Design review of the part built by this model. Coordinates are the model's own, in mm. A direction names the side the tool comes from. Coordinates: 2 decimals unless noted, no trailing zeros. Loops run counter-clockwise (first coordinate to the right, second up) from the corner with the lowest first, then second, coordinate; pieces in that order, holes last. Notation, with made-up numbers: M -21,2.25 L 30,2.25 A25 ccw 30,26.25 Z; hole C -13.75,83 d9. An arc over 180 degrees is marked long. Put each result on its own line as item: value. Start each with the question number.
(1) Clearance check with a flat-ended pin moving along its axis: pin 1 (4 mm diameter, centred on x = 39.5, z = 30, fed in from +Y). State where the tip first meets the part, or that it passes through.
(2) The part is to be moulded in two halves that separate along Y. For faces 3 (the cylindrical face through (0.49, 7.07, 28.5)), 4 (the flat face through (34.8, 0.3, 40)), 5 (the flat face through (36, 1, 20)), 6 (the cylindrical face through (0.5, 6.1, 8.8)), say which applies: +Y half, -Y half, draft (parallel to the pull), parting line (faces both ways), or undercut.
(3) For probe 1 along Y at (x, z) = (0.7, 10); probe 2 along Y at (x, z) = (16, 12.5), list the stretches that pass through material, from the lowest coordinate up. Write a range as [from, to].
(4) Take a section at B-B, the plane x = 30. Give the boundary of the cut face in (y, z).
(5) Take a section at A-A, the plane y = 7. Give the boundary of the cut face in (x, z).
(6) Take a section at D-D, the plane x = 10.5. Give the boundary of the cut face in (y, z).
(7) Take a section at C-C, the plane z = 33.5. Give the boundary of the cut face in (x, y), then the cut area to 3 significant figures.
(8) For faces 1 (the flat face through (1, 8, 20)), 2 (the flat face through (0, 8, 20)), list the 3-axis set-ups (+Z, -Z, +X, -X, +Y, -Y) from which the entire face can be reached by the end or side of a thin tool; tool diameter is ignored.
```python
from build123d import *

# Parameters (mm, degrees)
BOSS_EXTRUDE1_DEPTH = 40
SKETCH2_W           = 45
SKETCH2_H           = 3
CUT_EXTRUDE1_DEPTH  = 10
SKETCH3_R           = 1.5
CUT_EXTRUDE2_DEPTH  = 10


with BuildPart() as part:
    # Sketch1 → Boss-Extrude1 (new body)
    with BuildSketch(Plane.XY):
        Polygon((0, 0), (70, 0), (70, 1), (1, 1), (1, 15), (0, 15), align=None)
    extrude(amount=BOSS_EXTRUDE1_DEPTH)

    # Sketch2 → Cut-Extrude1 (cut)
    with BuildSketch(Plane(origin=(0, 1, 0), x_dir=(1, 0, 0), z_dir=(0, 1, 0))):
        with Locations((42.5, -8)):
            Rectangle(SKETCH2_W, SKETCH2_H)
        with Locations((42.5, -31)):
            Rectangle(SKETCH2_W, SKETCH2_H)
    extrude(amount=-CUT_EXTRUDE1_DEPTH, mode=Mode.SUBTRACT)

    # Sketch3 → Cut-Extrude2 (cut)
    with BuildSketch(Plane.ZY):
        with Locations((30, 7)):
            Circle(SKETCH3_R)
        with Locations((10, 7)):
            Circle(SKETCH3_R)
    extrude(amount=-CUT_EXTRUDE2_DEPTH, mode=Mode.SUBTRACT)


solid = part.part
```
Computed values:
1. pin 1: stops at y = 1
2. face 3: undercut
2. face 4: draft
2. face 5: +Y half
2. face 6: undercut
3. probe 1: y = [0, 5.5], [8.5, 15]
3. probe 2: y = [0, 1]
4. outline: M 0,0 L 1,0 L 1,6.5 L 0,6.5 Z; M 0,9.5 L 1,9.5 L 1,29.5 L 0,29.5 Z; M 0,32.5 L 1,32.5 L 1,40 L 0,40 Z
5. outline: M 0,0 L 1,0 L 1,8.5 L 0,8.5 Z; M 0,11.5 L 1,11.5 L 1,28.5 L 0,28.5 Z; M 0,31.5 L 1,31.5 L 1,40 L 0,40 Z
6. outline: M 0,0 L 1,0 L 1,40 L 0,40 Z
7. outline: M 0,0 L 70,0 L 70,1 L 1,1 L 1,15 L 0,15 Z
7. area: 84.0 mm^2
8. face 1: +Z, -Z, +X, +Y
8. face 2: +Z, -Z, -X, +Y, -Y
